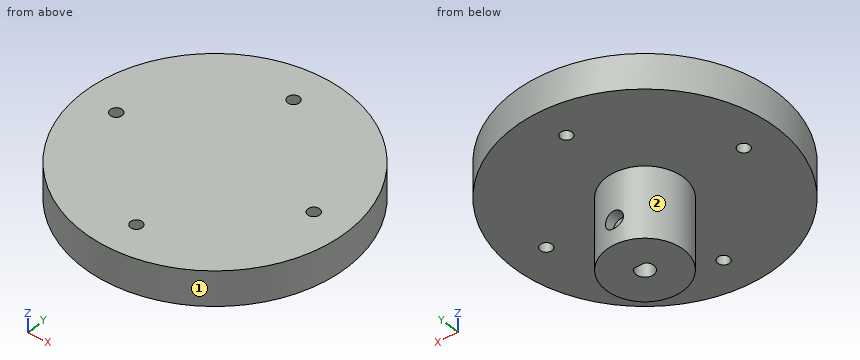
Autodesk Fusion 360 part; units mm, degrees
sketch "Sketch1" plane through (0, 0, 0) normal (0, 0, 1) x (1, 0, 0)
  circle A0 centre (0, 0) radius 37.5
  dimension "d1" = 75
extrude "Extrude1" add sketch "Sketch1" along normal blind 10
sketch "Sketch2" plane through (0, 0, 0) normal (0, 0, -1) x (1, 0, 0)
  circle A0 centre (0, 0) radius 37.5
  circle A1 centre (0, 0) radius 10.985
  dimension "d4" = 21.97
extrude "Extrude2" add sketch "Sketch2" along normal blind 20.3 contours A1
sketch "Sketch3" plane through (0, 0, -20.3) normal (0, 0, -1) x (1, 0, 0)
  circle A0 centre (0, 0) radius 10.985
  circle A1 centre (0, 0) radius 2.5
  dimension "d7" = 5
extrude "Extrude3" cut sketch "Sketch3" against normal blind 20.3 contours A1
sketch "Sketch5" plane through (0, 0, -20.3) normal (0, 0, -1) x (1, 0, 0)
  circle A0 centre (0, 0) radius 2.5
  circle A1 centre (0, 0) radius 10.985
  line L0 (0, -1.992) -> (1.5106, -1.992)
  line L1 (0, -1.992) -> (-1.5106, -1.992)
  circle A2 centre (0, 0) radius 2.5
extrude "Extrude4" add sketch "Sketch5" against normal blind 20.3 contours A0 L0 L1 A2 picked at (0, -2.3263)
sketch "Sketch6" plane through (0, 1.992, 0) normal (0, -1, 0) x (1, 0, 0)
  line L0 (-1.5106, -20.3) -> (1.5106, -20.3)
  line L1 (1.5106, -20.3) -> (1.5106, 0)
  line L2 (1.5106, 0) -> (-1.5106, 0)
  line L3 (-1.5106, 0) -> (-1.5106, -20.3)
sketch "Sketch7" plane through (0, 0, -20.3) normal (0, 0, -1) x (1, 0, 0)
  arc A0 (1.5106, -1.992) -> (-1.5106, -1.992) centre (0, 0) ccw
  line L0 (1.5106, -1.992) -> (-1.5106, -1.992)
  circle A1 centre (0, 0) radius 10.985
hole "Hole1" at (0, 10.985, -13.2045) direction (0, -1, 0) diameter 2.175 depth 50 tip angle 180 counterbore diameter 5 counterbore depth 3
sketch "Sketch8" plane through (0, 0, 10) normal (0, 0, 1) x (-1, 0, 0)
  circle A0 centre (0, 0) radius 37.5
sketch "Sketch9" plane through (0, 0, 10) normal (0, 0, 1) x (-1, 0, 0)
  circle A0 centre (0, 0) radius 37.5
  line L0 (-0.0392, -37.5) -> (-0.0278, -27.5)
  line L1 (37.5, -0.0392) -> (27.5, -0.0278)
  line L2 (0.0392, 37.5) -> (0.0278, 27.5)
  line L3 (-37.5, 0.0392) -> (-27.5, 0.0278)
  dimension "d19" = 10
  dimension "d21" = 360
hole "Hole2" at (0.0278, 27.5, 10) at (27.5, -0.0278, 10) at (-0.0278, -27.5, 10) at (-27.5, 0.0278, 10) direction (0, 0, -1) diameter 3.332 depth 50 tip angle 180
component "6627T91_Stepper Motor" placed x (1, 0, 0) y (0, 1, 0) z (0, 0, 1) at (52.5447, 49.4652, -3.0795)
Verification items for the finished model (mm, model axes). Face numbers are marked on the shaded views. A direction names the side the tool comes from. Coordinates: 2 decimals unless noted, no trailing zeros. Loops run counter-clockwise (first coordinate to the right, second up) from the corner with the lowest first, then second, coordinate; pieces in that order, holes last. Notation, with made-up numbers: (19.5, 24.5) -> (50.5, 24.5) arc R29 ccw to (50.5, 54.5) -> close; hole circle Ø8 at (30, 33). An arc over 180 degrees is marked (long way). Answer in a Markdown table with one row per item. Add a question column.
1. Material ranges on probe 1 along X at (y, z) = (0, -4.5) (3 decimals); probe 2 along Z at (x, y) = (0, 6.1); probe 3 along X at (y, z) = (-1, 8), recorded low to high. Write a range as [from, to].
2. Access from +Z, -Z, +X, -X, +Y, -Y to the whole of each face (thin tool, end or side, straight path). Record for the marked faces 1 and 2.
3. Depth check by flat-ended pin: P1, Ø12, axis at y = 26.5, z = -8.5, coming from the -X side; P2, Ø2.5, axis at x = 0, z = -13.2, coming from the +Y side (3 decimals); P3, Ø3, axis at x = 0, y = -25.5, coming from the -Z side; P4, Ø5, axis at x = 7.5, z = -6, coming from the +Y side. Enter the tip coordinate at first touch or a pass-through.
4. Section check A-A, the plane y = 27.5. Enter the section's corners in (x, z), then the cut area to 3 significant figures.
5. Section check C-C, the plane y = 0. Enter the section's corners in (x, z) (3 decimals), then the cut area to 3 significant figures.
6. Section check D-D, the plane z = -17.5. Enter the section's corners in (x, y) (3 decimals).
Derived:
| question | item | result |
|---|---|---|
| 1 | probe 1 | x = [-10.985, -2.5], [2.5, 10.985] |
| 1 | probe 2 | z = [-20.3, -14.29], [-12.12, 10] |
| 1 | probe 3 | x = [-37.49, -28.81], [-26.19, 26.15], [28.85, 37.49] |
| 2 | face 1 | +Z, -Z |
| 2 | face 2 | -Z |
| 3 | P1 | passes through |
| 3 | P2 | stops at y = 7.985 |
| 3 | P3 | stops at z = 0 |
| 3 | P4 | stops at y = 9.78 |
| 4 | outline | (-25.5, 0) -> (-1.64, 0) -> (-1.64, 10) -> (-25.5, 10) -> close; (1.69, 0) -> (25.5, 0) -> (25.5, 10) -> (1.69, 10) -> close |
| 4 | area | 477 mm² |
| 5 | outline | (-37.5, 0) -> (-29.166, 0) -> (-29.166, 10) -> (-37.5, 10) -> close; (-25.834, 0) -> (-10.985, 0) -> (-10.985, -20.3) -> (-2.5, -20.3) -> (-2.5, 0) -> (2.5, 0) -> (2.5, -20.3) -> (10.985, -20.3) -> (10.985, 0) -> (25.834, 0) -> (25.834, 10) -> (-25.834, 10) -> close; (29.166, 0) -> (37.5, 0) -> (37.5, 10) -> (29.166, 10) -> close |
| 5 | area | 1,030 mm² |
| 6 | outline | circle Ø21.97 at (0, 0); hole (-1.511, 1.992) arc R2.5 ccw (long way) to (1.511, 1.992) -> close |
